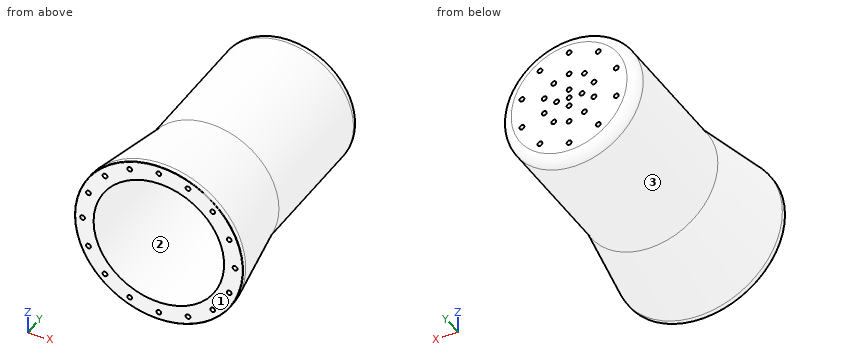
```python
from build123d import *

# Parameters (mm, degrees)
SKETCH2_R          = 2.3
CUT_EXTRUDE1_DEPTH = 10
SKETCH4_R          = 2.3
CUT_EXTRUDE2_DEPTH = 6.25
CHAMFER3_SIZE      = 20
FILLET10_R         = 10
FILLET15_R         = 0.5


with BuildPart() as part:
    # Sketch1 one side → Revolve1 (revolve)
    with BuildSketch(Plane.XY, mode=Mode.PRIVATE) as revolve1_sk:
        Polygon((80.5, 5), (65.5, 90.069227294), (65.5, 230), (0, 230), (0, 220), (62.5, 220), (62.5, 0), (80.5, 0), align=None)
    revolve(revolve1_sk.sketch.rotate(Axis((0, 230, 0), (0, -1, 0)), 180), axis=Axis((0, 230, 0), (0, -1, 0)))

    # Sketch2 → Cut-Extrude1 (cut)
    with BuildSketch(Plane.XZ):
        with Locations((73, 0)):
            Circle(SKETCH2_R)
        with Locations((67.443205873, -27.935890563)):
            Circle(SKETCH2_R)
        with Locations((51.618795027, -51.618795027)):
            Circle(SKETCH2_R)
        with Locations((27.935890563, -67.443205873)):
            Circle(SKETCH2_R)
        with Locations((0, -73)):
            Circle(SKETCH2_R)
        with Locations((-27.935890563, -67.443205873)):
            Circle(SKETCH2_R)
        with Locations((-51.618795027, -51.618795027)):
            Circle(SKETCH2_R)
        with Locations((-67.443205873, -27.935890563)):
            Circle(SKETCH2_R)
        with Locations((-73, 0)):
            Circle(SKETCH2_R)
        with Locations((-67.443205873, 27.935890563)):
            Circle(SKETCH2_R)
        with Locations((-51.618795027, 51.618795027)):
            Circle(SKETCH2_R)
        with Locations((-27.935890563, 67.443205873)):
            Circle(SKETCH2_R)
        with Locations((0, 73)):
            Circle(SKETCH2_R)
        with Locations((27.935890563, 67.443205873)):
            Circle(SKETCH2_R)
        with Locations((51.618795027, 51.618795027)):
            Circle(SKETCH2_R)
        with Locations((67.443205873, 27.935890563)):
            Circle(SKETCH2_R)
    extrude(amount=-CUT_EXTRUDE1_DEPTH, mode=Mode.SUBTRACT)

    # Sketch4 → Cut-Extrude2 (cut)
    with BuildSketch(Plane(origin=(0, 230, 0), x_dir=(1, 0, 0), z_dir=(0, 1, 0))):
        with Locations(Location((0, 47.5, 0), (0, 0, 180))):
            Circle(SKETCH4_R)
        with Locations(Location((0, 25, 0), (0, 0, 180))):
            Circle(SKETCH4_R)
        with Locations(Location((27.919799484, 38.428307233, 0), (0, 0, 180))):
            Circle(SKETCH4_R)
        with Locations(Location((14.694631307, 20.225424859, 0), (0, 0, 180))):
            Circle(SKETCH4_R)
        with Locations(Location((45.175184524, 14.678307233, 0), (0, 0, 180))):
            Circle(SKETCH4_R)
        with Locations(Location((23.776412907, 7.725424859, 0), (0, 0, 180))):
            Circle(SKETCH4_R)
        with Locations(Location((45.175184524, -14.678307233, 0), (0, 0, 180))):
            Circle(SKETCH4_R)
        with Locations(Location((23.776412907, -7.725424859, 0), (0, 0, 180))):
            Circle(SKETCH4_R)
        with Locations(Location((27.919799484, -38.428307233, 0), (0, 0, 180))):
            Circle(SKETCH4_R)
        with Locations(Location((14.694631307, -20.225424859, 0), (0, 0, 180))):
            Circle(SKETCH4_R)
        with Locations(Location((0, -47.5, 0), (0, 0, 180))):
            Circle(SKETCH4_R)
        with Locations(Location((0, -25, 0), (0, 0, 180))):
            Circle(SKETCH4_R)
        with Locations(Location((-27.919799484, -38.428307233, 0), (0, 0, 180))):
            Circle(SKETCH4_R)
        with Locations(Location((-14.694631307, -20.225424859, 0), (0, 0, 180))):
            Circle(SKETCH4_R)
        with Locations(Location((-45.175184524, -14.678307233, 0), (0, 0, 180))):
            Circle(SKETCH4_R)
        with Locations(Location((-23.776412907, -7.725424859, 0), (0, 0, 180))):
            Circle(SKETCH4_R)
        with Locations(Location((-45.175184524, 14.678307233, 0), (0, 0, 180))):
            Circle(SKETCH4_R)
        with Locations(Location((-23.776412907, 7.725424859, 0), (0, 0, 180))):
            Circle(SKETCH4_R)
        with Locations(Location((-27.919799484, 38.428307233, 0), (0, 0, 180))):
            Circle(SKETCH4_R)
        with Locations(Location((-14.694631307, 20.225424859, 0), (0, 0, 180))):
            Circle(SKETCH4_R)
        with Locations(Location((0, 0, 0), (0, 0, 180))):
            Circle(SKETCH4_R)
        with Locations(Location((11.997484215, 0, 0), (0, 0, 180))):
            Circle(SKETCH4_R)
        with Locations(Location((-12.341543393, 0, 0), (0, 0, 180))):
            Circle(SKETCH4_R)
        with Locations(Location((0, 8.5, 0), (0, 0, 180))):
            Circle(SKETCH4_R)
        with Locations(Location((0, -8.5, 0), (0, 0, 180))):
            Circle(SKETCH4_R)
    extrude(amount=-CUT_EXTRUDE2_DEPTH, mode=Mode.SUBTRACT)

    # Chamfer3
    chamfer3_edges = [part.edges().sort_by_distance(p)[0] for p in [
        (62.5, 220, 0),
    ]]
    chamfer(chamfer3_edges, length=CHAMFER3_SIZE)

    # Fillet10
    fillet10_edges = [part.edges().sort_by_distance(p)[0] for p in [
        (65.5, 230, 0),
    ]]
    fillet(fillet10_edges, radius=FILLET10_R)

    # Fillet15
    fillet15_edges = [part.edges().sort_by_distance(p)[0] for p in [
        (80.5, 0, 0),
    ]]
    fillet(fillet15_edges, radius=FILLET15_R)


solid = part.part
```
Part model, mm, in its own coordinate system. Face numbers are marked on the shaded views. Round coordinates to 2 decimals unless told otherwise and drop trailing zeros. Write each loop counter-clockwise with the first axis right and the second up, starting at its lowest first coordinate (ties: lowest second). Pieces come first, ordered by that corner, then holes. Notation, with made-up numbers: (88.5, -11) -> (120.5, -11) arc R14 cw to (120.5, 8) -> close; hole circle Ø2 at (17.25, 61.25). An arc over 180 degrees is marked (long way). Return JSON: item names as keys, results as strings. Group by question number.
Q1. Pin check, flat tips, straight feed: pin 1 (12 mm diameter, centred on y = 115.5, z = 34.5, fed in from +X); pin 2 (5 mm diameter, centred on x = -14.5, z = 20.5, fed in from +Y); pin 3 (1.4 mm diameter, centred on x = 46, z = -13.5, fed in from +Y); pin 4 (1 mm diameter, centred on x = 1, y = 200, fed in from -Z). Stop position of each tip, or through.
Q2. Mould opens along X. For the marked faces 1, 2 and 3 say: pulls with the +X half, pulls with the -X half, needs draft (parallel to the pull), parting line crosses it, or undercut.
Q3. Saw through at A-A on y = 131.5. Write the cut outline in (x, z), plus the area to 3 significant figures.
Q4. Probe L1, parallel to Y at x = -12, z = 30; L2, parallel to Z at x = -32.5, y = 35; L3, parallel to Z at x = -13.5, y = 124. List the from-to ranges inside material, lowest first. Write a range as [from, to].
Answer:
{
 "1": {"pin 1": "x = 58.97", "pin 2": "y = 230", "pin 3": "y = 223.75", "pin 4": "z = -65.5"},
 "2": {"face 1": "needs draft", "face 2": "undercut", "face 3": "parting line crosses it"},
 "3": {"outline": "circle Ø131 at (0, 0); hole circle Ø125 at (0, 0)", "area": "1,210 mm2"},
 "4": {"L1": "[220, 230]", "L2": "[-67.83, -53.39], [53.39, 67.83]", "L3": "[-64.09, -61.02], [61.02, 64.09]"}
}
